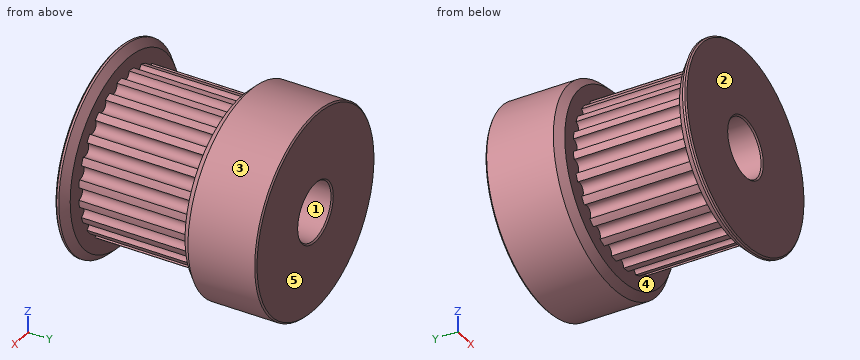
from build123d import *

# Parameters (mm, degrees)
F0_R     = 11
F1_DEPTH = 8
F2_R     = 14
F3_DEPTH = 1.5
F4_R     = 14
F5_DEPTH = 10.5
F6_R     = 4
F7_DEPTH = 28.001
F8_R     = 0.9
F9_DEPTH = 16
F10_SIZE = 1
F11_SIZE = 0.2


with BuildPart() as f1:
    # F0 (on Front) → F1 (new body, symmetric)
    with BuildSketch(Plane.XZ):
        Circle(F0_R)
    extrude(amount=F1_DEPTH, both=True)

    # F2 (on face) → F3 (join)
    with BuildSketch(Plane.XZ.offset(8)):
        Circle(F2_R)
    extrude(amount=F3_DEPTH)

    # F4 (on face) → F5 (join)
    with BuildSketch(Plane(origin=(0, 8, 0), x_dir=(-1, 0, 0), z_dir=(0, 1, 0))):
        Circle(F4_R)
    extrude(amount=F5_DEPTH)

    # F6 (on face) → F7 (cut, through all)
    with BuildSketch(Plane(origin=(0, 18.5, 0), x_dir=(-1, 0, 0), z_dir=(0, 1, 0))):
        Circle(F6_R)
    extrude(amount=-F7_DEPTH, mode=Mode.SUBTRACT)

    # F8 (on face) → F9 (cut, through all)
    with BuildSketch(Plane.XZ.offset(-8)):
        with Locations((0, 11)):
            Circle(F8_R)
        with Locations((-2.8470094961, 10.6251840892)):
            Circle(F8_R)
        with Locations((-5.5, 9.5262794416)):
            Circle(F8_R)
        with Locations((-7.7781745931, 7.7781745931)):
            Circle(F8_R)
        with Locations((-9.5262794416, 5.5)):
            Circle(F8_R)
        with Locations((-10.6251840892, 2.8470094961)):
            Circle(F8_R)
        with Locations((-11, 0)):
            Circle(F8_R)
        with Locations((-10.6251840892, -2.8470094961)):
            Circle(F8_R)
        with Locations((-9.5262794416, -5.5)):
            Circle(F8_R)
        with Locations((-7.7781745931, -7.7781745931)):
            Circle(F8_R)
        with Locations((-5.5, -9.5262794416)):
            Circle(F8_R)
        with Locations((-2.8470094961, -10.6251840892)):
            Circle(F8_R)
        with Locations((0, -11)):
            Circle(F8_R)
        with Locations((2.8470094961, -10.6251840892)):
            Circle(F8_R)
        with Locations((5.5, -9.5262794416)):
            Circle(F8_R)
        with Locations((7.7781745931, -7.7781745931)):
            Circle(F8_R)
        with Locations((9.5262794416, -5.5)):
            Circle(F8_R)
        with Locations((10.6251840892, -2.8470094961)):
            Circle(F8_R)
        with Locations((11, 0)):
            Circle(F8_R)
        with Locations((10.6251840892, 2.8470094961)):
            Circle(F8_R)
        with Locations((9.5262794416, 5.5)):
            Circle(F8_R)
        with Locations((7.7781745931, 7.7781745931)):
            Circle(F8_R)
        with Locations((5.5, 9.5262794416)):
            Circle(F8_R)
        with Locations((2.8470094961, 10.6251840892)):
            Circle(F8_R)
    extrude(amount=F9_DEPTH, mode=Mode.SUBTRACT)

    # F10
    f10_edges = [f1.edges().sort_by_distance(p)[0] for p in [
        (-14, -8, 0),
        (14, 8, 0),
    ]]
    chamfer(f10_edges, length=F10_SIZE)

    # F11
    f11_edges = [f1.edges().sort_by_distance(p)[0] for p in [
        (-14, -9.5, 0),
        (4, -9.5, 0),
        (14, 18.5, 0),
        (4, 18.5, 0),
    ]]
    chamfer(f11_edges, length=F11_SIZE)


solid = f1.part
Can you work these out from the model? Positions are in its coordinate system, mm. Face numbers are marked on the shaded views. A direction names the side the tool comes from. Round coordinates to 2 decimals unless told otherwise and drop trailing zeros. Order: outer loops, then holes, each group sorted by start corner. A loop starts at its lowest first (then second) coordinate and runs counter-clockwise, first axis right, second up. Notation, with made-up numbers: M 17,77.25 L 47,77.25 A27 ccw 47,102.25 Z; hole C 28,19 d1. An arc over 180 degrees is marked long. Use a Markdown table: item, result.
1) I'm going to push flat-ended pins straight in: P1, Ø13, axis at x = 0, z = -0.5, coming from the +Y side; P2, Ø1.5, axis at y = -3, z = -7.5, coming from the +X side; P3, Ø4, axis at y = 8.5, z = 11, coming from the -X side; P4, Ø1.5, axis at y = -4.5, z = -10.5, coming from the -X side. Where does each tip first touch, or does it pass through?
Geometry says:
| item | result |
|---|---|
| P1 | stops at y = 18.5 |
| P2 | stops at x = 8.69 |
| P3 | stops at x = -10.67 |
| P4 | stops at x = -4.7 |
2) If I drill on line 1 along Y through (x, z) = (3.75, 10.75); line 2 along X through (y, z) = (-3.25, 8.75); line 3 along Z through (x, y) = (0, 8.75), over which ranges is the centre line in solid material (lowest first)?
Geometry says:
| item | result |
|---|---|
| line 1 | y = -9.5 to -8, 8 to 18.5 |
| line 2 | x = -6.67 to -5.96, -5.04 to 5.04, 5.96 to 6.67 |
| line 3 | z = -13.75 to -4, 4 to 13.75 |
3) Imagine slicing it at A-A (x = 0). List the corners of the cut face in (y, z) for me.
Geometry says:
| item | result |
|---|---|
| outline | M -9.5,-13.8 L -9.3,-14 L -9,-14 L -8,-13 L -8,-10.1 L 8,-10.1 L 8,-13 L 9,-14 L 18.3,-14 L 18.5,-13.8 L 18.5,-4.2 L 18.3,-4 L -9.3,-4 L -9.5,-4.2 Z; M -9.5,4.2 L -9.3,4 L 18.3,4 L 18.5,4.2 L 18.5,13.8 L 18.3,14 L 9,14 L 8,13 L 8,10.1 L -8,10.1 L -8,13 L -9,14 L -9.3,14 L -9.5,13.8 Z |
4) Imagine slicing it at B-B (y = 11.75). List the corners of the cut face in (x, z) for me, then the cut area to 3 significant figures.
Geometry says:
| item | result |
|---|---|
| outline | C 0,0 d28; hole C 0,0 d8 |
| area | 565 mm² |
5) On a 3-axis mill with a long thin cutter (end or side, diameter ignored), from which of +Z, -Z, +X, -X, +Y, -Y can I reach the whole of each face in a straight line? I mean the marked faces 4 and 5. Say none if no direction works.
Geometry says:
| item | result |
|---|---|
| face 4 | none |
| face 5 | +Z, -Z, +X, -X, +Y |
6) If we mould it in two halves opening along X, with no side actions, what happens to the marked faces 1, 2 and 3? For each: +X half, -X half, draft (parallel to the pull), parting line (faces both ways), or undercut.
Geometry says:
| item | result |
|---|---|
| face 1 | undercut |
| face 2 | draft |
| face 3 | parting line |
